Geometry: see drawing. Coordinates: mm, zero at the bounding-box minimum. A direction names the side the tool comes from. Coordinates: 2 decimals unless noted, no trailing zeros. Loops run counter-clockwise (first coordinate to the right, second up) from the corner with the lowest first, then second, coordinate; pieces in that order, holes last. Notation, with made-up numbers: M -38,69.5 L 13,69.5 A34 cw 13,103.5 Z; hole C 0.5,68 d11. An arc over 180 degrees is marked long. One line per question, with ' | ' between items. Start each with the question number.
1. Section query C-C, the plane x = 7.5. Output: boundary loops of the cut face in (y, z), and give its area (3 significant figures).
2. Ray query, probe 1 along X at (y, z) = (128.5, 10); probe 2 along Z at (x, y) = (1.25, 130); probe 3 along Y at (x, z) = (3.5, 11). Return the intervals inside material, ascending.
3. Pin query (flat end, axial travel): P1, Ø1.5, axis at x = 11, y = 76.5, coming from the -Z side; P2, Ø4.5, axis at x = 8, y = 102.5, coming from the -Z side; P3, Ø3, axis at y = 39.5, z = 1.5, coming from the -X side; P4, Ø1, axis at y = 70, z = 10, coming from the +X side. Return the tip coordinate at first contact, or that it passes through.
4. Section query A-A, the plane y = 45. Output: boundary loops of the cut face in (x, z), and give its area (3 significant figures).
5. Access query for the marked faces 1, 2, 3, 4 and 5. Directions: +Z, -Z, +X, -X, +Y, -Y. A direction counts if a zero-diameter tool reaches every point of the face in a straight line with its end or side. Return the directions, or none.
6. Section query D-D, the plane y = 13.5. Output: boundary loops of the cut face in (x, z).
7. Section query B-B, the plane z = 8. Output: boundary loops of the cut face in (x, y).
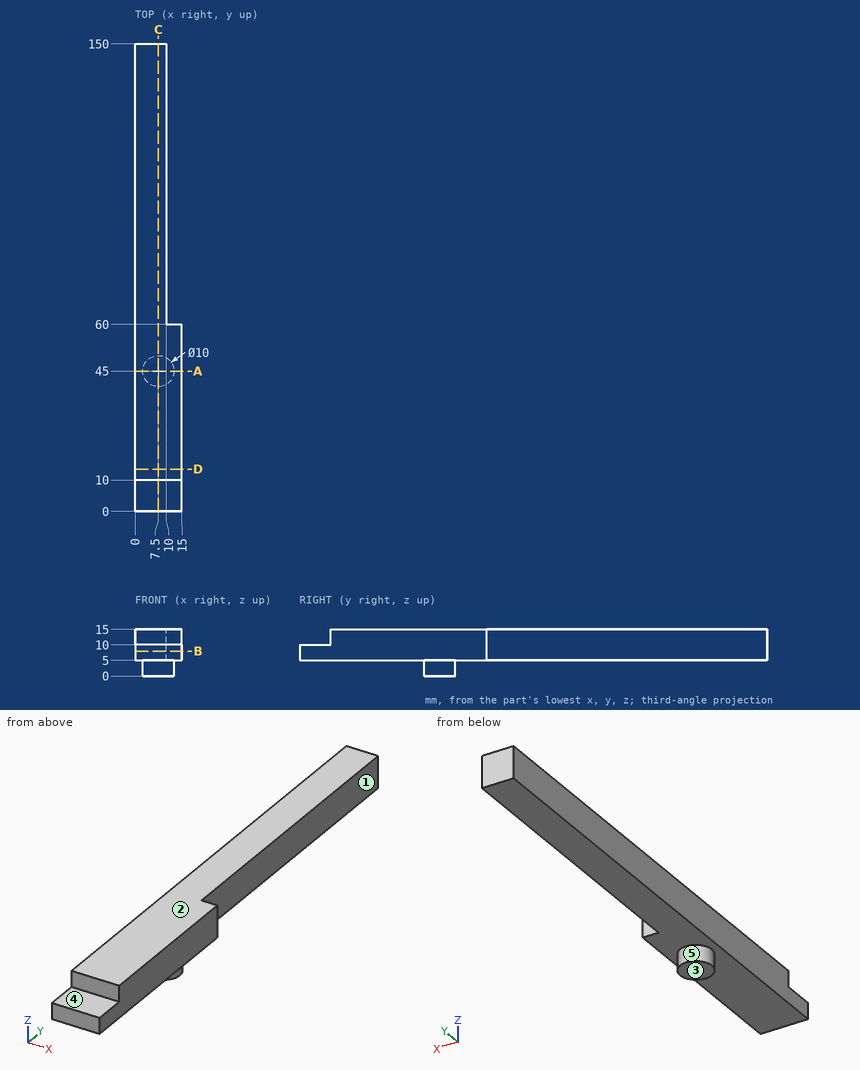
Taken from the geometry:
1) outline: M 0,5 L 40,5 L 40,0 L 50,0 L 50,5 L 150,5 L 150,15 L 10,15 L 10,10 L 0,10 Z | area: 1,500 mm^2
2) probe 1: 0 to 10 | probe 2: 5 to 15 | probe 3: 10 to 150
3) P1: through | P2: z = 5 | P3: x = 4.5 | P4: x = 10
4) outline: M 0,5 L 2.5,5 L 2.5,0 L 12.5,0 L 12.5,5 L 15,5 L 15,15 L 0,15 Z | area: 200 mm^2
5) face 1: +Z, -Z, +X, +Y | face 2: +Z, +X, -X, +Y, -Y | face 3: -Z, +X, -X, +Y, -Y | face 4: +Z, +X, -X, -Y | face 5: -Z
6) outline: M 0,5 L 15,5 L 15,15 L 0,15 Z
7) outline: M 0,0 L 15,0 L 15,60 L 10,60 L 10,150 L 0,150 Z
